from build123d import *

# Parameters (mm, degrees)
F0_W     = 88.869118
F0_H     = 83.88424
F1_DEPTH = 77.4465
F2_R     = 34.214066
F3_R     = 11.016675
F4_DEPTH = 25.4


with BuildPart() as f1:
    # F0 (on Front) → F1 (new body)
    with BuildSketch(Plane.XZ):
        Rectangle(F0_W, F0_H)
    extrude(amount=F1_DEPTH)

    # F2
    f2_edges = [f1.edges().sort_by_distance(p)[0] for p in [
        (-44.434559, -38.72325, 41.94212),
    ]]
    fillet(f2_edges, radius=F2_R)

    # F3 (on face) → F4 (join)
    with BuildSketch(Plane.XZ.offset(77.4465)):
        with Locations((-10.220493, 7.728054)):
            Circle(F3_R)
        with Locations((32.314323, -24.676727)):
            Circle(F3_R)
    extrude(amount=F4_DEPTH)


solid = f1.part
Geometry: final body of the model. Coordinates: model frame, mm. A direction names the side the tool comes from. Round coordinates to 2 decimals unless told otherwise and drop trailing zeros. Loops run counter-clockwise (first coordinate to the right, second up) from the corner with the lowest first, then second, coordinate; pieces in that order, holes last.
Q1. Pin query (flat end, axial travel): P1, Ø6, axis at x = -35, z = -30.5, coming from the -Y side; P2, Ø6, axis at x = 21.5, y = -80.5, coming from the -Z side; P3, Ø10, axis at y = -77, z = 26, coming from the -X side. Return the tip coordinate at first contact, or that it passes through.
Q2. Section D-D on x = 16.5. Return loops of the section in (y, z), plus the area to 3 significant figures.
Q3. Section B-B on x = -5. Return loops of the section in (y, z), plus the area to 3 significant figures.
Q4. Section C-C on z = -15. Return loops of the section in (x, y), plus the area to 3 significant figures.
Q5. Access query for faces 1 (the cylindrical face through (42.822, -89.969, -21.368)), 2 (the flat face through (-1, -38, -41.942)). Directions: +Z, -Z, +X, -X, +Y, -Y. A direction counts if a zero-diameter tool reaches every point of the face in a straight line with its end or side. Return the directions, or none.
Q6. Section A-A on y = -75.5. Return loops of the section in (x, z), plus the area to 3 significant figures.
Q7. Material intervals for L1, parallel to Y at x = -2, z = -20.5; L2, parallel to Z at x = -26.5, y = -49; L3, parallel to X at y = -93, z = -28.5, sorted ascending.
Evaluation:
1. P1: stops at y = -77.45
1. P2: stops at z = -32.44
1. P3: stops at x = -41.76
2. outline: (-77.45, -41.94) - (0, -41.94) - (0, 41.94) - (-77.45, 41.94) - close
2. area: 6,500 mm2
3. outline: (-102.85, -1.97) - (-77.45, -1.97) - (-77.45, -41.94) - (0, -41.94) - (0, 41.94) - (-77.45, 41.94) - (-77.45, 17.43) - (-102.85, 17.43) - close
3. area: 6,990 mm2
4. outline: (-44.43, -77.45) - (27.05, -77.45) - (27.05, -102.85) - (37.58, -102.85) - (37.58, -77.45) - (44.43, -77.45) - (44.43, 0) - (-44.43, 0) - close
4. area: 7,150 mm2
5. face 1: -Y
5. face 2: -Z, +X, -X, +Y, -Y
6. outline: (-44.43, -41.94) - (44.43, -41.94) - (44.43, 41.94) - (-10.22, 41.94) arc R34.21 ccw to (-44.43, 7.73) - close
6. area: 7,200 mm2
7. L1: y = -77.45 to 0
7. L2: z = -41.94 to 37.82
7. L3: x = 21.98 to 42.65
